Check sheet for the modelled part. Datum: model origin and axes. Units: mm. Face numbers are marked on the shaded views. A direction names the side the tool comes from. Give positions to 0.01 mm unless a question says otherwise; leave off trailing zeros. Write each loop counter-clockwise with the first axis right and the second up, starting at its lowest first coordinate (ties: lowest second). Pieces come first, ordered by that corner, then holes. Notation, with made-up numbers: (-29, 43) -> (-6, 43) arc R14 cw to (-6, 64) -> close; hole circle Ø4 at (59.25, -23.5). An arc over 180 degrees is marked (long way). Answer as a JSON object with one key per item and string values.
from build123d import *

# Parameters (mm, degrees)
SKETCH1_W                                         = 101.6
SKETCH1_H                                         = 100.0125
BOSS_EXTRUDE1_DEPTH                               = 10.16
CBORE_FOR_5_16_SOCKET_HEAD_CAP_SCREW1_D           = 8.2042
CBORE_FOR_5_16_SOCKET_HEAD_CAP_SCREW1_CBORE_D     = 13.49502
CBORE_FOR_5_16_SOCKET_HEAD_CAP_SCREW1_CBORE_DEPTH = 7.9375
SKETCH4_R                                         = 30.1625
BOSS_EXTRUDE2_DEPTH                               = 2.54
CBORE_FOR_3_8_SOCKET_HEAD_CAP_SCREW1_D            = 9.8044
CBORE_FOR_3_8_SOCKET_HEAD_CAP_SCREW1_CBORE_D      = 15.875
CBORE_FOR_3_8_SOCKET_HEAD_CAP_SCREW1_CBORE_DEPTH  = 9.525
FILLET1_R                                         = 2.54


with BuildPart() as part:
    # Sketch1 → Boss-Extrude1 (new body)
    with BuildSketch(Plane.XY):
        with Locations((50.8, 50.00625)):
            Rectangle(SKETCH1_W, SKETCH1_H)
    extrude(amount=BOSS_EXTRUDE1_DEPTH)

    # CBORE for 5/16 Socket Head Cap Screw1 (through all)
    with Locations(Plane.XY.offset(10.16)):
        with Locations((88.9, 8.73125), (88.9, 91.28125), (12.7, 8.73125), (12.7, 91.28125)):
            CounterBoreHole(CBORE_FOR_5_16_SOCKET_HEAD_CAP_SCREW1_D / 2, CBORE_FOR_5_16_SOCKET_HEAD_CAP_SCREW1_CBORE_D / 2, CBORE_FOR_5_16_SOCKET_HEAD_CAP_SCREW1_CBORE_DEPTH)

    # Sketch4 → Boss-Extrude2 (add)
    with BuildSketch(Plane.XY.offset(10.16)):
        with Locations(Location((50.8, 50.00625, 0), (0, 0, 180))):
            Circle(SKETCH4_R)
    extrude(amount=BOSS_EXTRUDE2_DEPTH)

    # CBORE for 3/8 Socket Head Cap Screw1 (through all)
    with Locations(Plane(origin=(0, 0, 0), x_dir=(-1, 0, 0), z_dir=(0, 0, -1))):
        with Locations((-50.8, 50.00625)):
            CounterBoreHole(CBORE_FOR_3_8_SOCKET_HEAD_CAP_SCREW1_D / 2, CBORE_FOR_3_8_SOCKET_HEAD_CAP_SCREW1_CBORE_D / 2, CBORE_FOR_3_8_SOCKET_HEAD_CAP_SCREW1_CBORE_DEPTH)

    # Fillet1
    fillet1_edges = [part.edges().sort_by_distance(p)[0] for p in [
        (0, 100.0125, 5.08),
        (101.6, 100.0125, 5.08),
        (101.6, 0, 5.08),
        (0, 0, 5.08),
    ]]
    fillet(fillet1_edges, radius=FILLET1_R)


solid = part.part
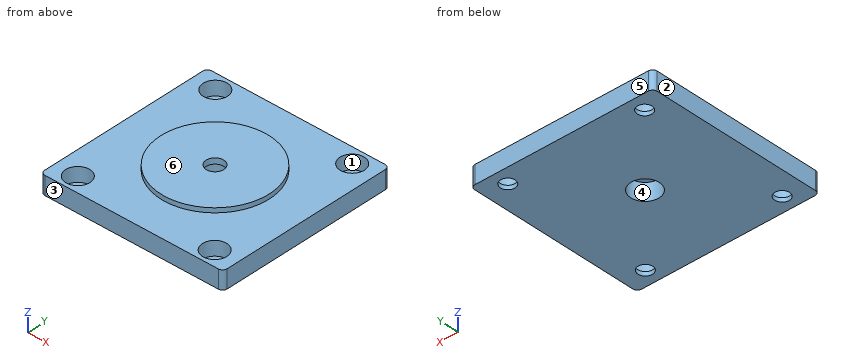
1. Scan lines: L1, parallel to Y at x = 88.9, z = 0.9; L2, parallel to Y at x = 88.9, z = 5.25; L3, parallel to Z at x = 27, y = 77. Record each from-to range of solid material in increasing order. Write a range as [from, to].
Determined:
{"L1": "[0, 4.63], [12.83, 87.18], [95.38, 100.01]", "L2": "[0, 1.98], [15.48, 84.53], [98.03, 100.01]", "L3": "[0, 10.16]"}
2. Mould release check, pull along Y, two halves, no side actions. Record for the marked faces 3, 4, 5 and 6: released by +Y, released by -Y, zero draft, split by the parting line, or undercut.
Determined:
{"face 3": "released by -Y", "face 4": "undercut", "face 5": "released by +Y", "face 6": "zero draft"}
3. Access from +Z, -Z, +X, -X, +Y, -Y to the whole of each face (thin tool, end or side, straight path). Record for the marked faces 1 and 2.
Determined:
{"face 1": "+Z", "face 2": "+Z, -Z, -X, +Y, -Y"}
4. Sectioned sample at B-B, the plane x = 12.7. Enter the section's corners in (y, z), plus the area to 3 significant figures.
Determined:
{"outline": "(0, 0) -> (4.63, 0) -> (4.63, 2.22) -> (1.98, 2.22) -> (1.98, 10.16) -> (0, 10.16) -> close; (12.83, 0) -> (87.18, 0) -> (87.18, 2.22) -> (84.53, 2.22) -> (84.53, 10.16) -> (15.48, 10.16) -> (15.48, 2.22) -> (12.83, 2.22) -> close; (95.38, 0) -> (100.01, 0) -> (100.01, 10.16) -> (98.03, 10.16) -> (98.03, 2.22) -> (95.38, 2.22) -> close", "area": "765 mm^2"}
5. Sectioned sample at A-A, the plane x = 50.8. Enter the section's corners in (y, z) (1 decimal), plus the area to 3 significant figures.
Determined:
{"outline": "(0, 0) -> (42.1, 0) -> (42.1, 9.5) -> (45.1, 9.5) -> (45.1, 12.7) -> (19.8, 12.7) -> (19.8, 10.2) -> (0, 10.2) -> close; (54.9, 9.5) -> (57.9, 9.5) -> (57.9, 0) -> (100, 0) -> (100, 10.2) -> (80.2, 10.2) -> (80.2, 12.7) -> (54.9, 12.7) -> close", "area": "987 mm^2"}
6. Sectioned sample at D-D, the plane z = 5. Enter the section's corners in (x, y) (1 decimal).
Determined:
{"outline": "(0, 2.5) arc R2.5 ccw to (2.5, 0) -> (99.1, 0) arc R2.5 ccw to (101.6, 2.5) -> (101.6, 97.5) arc R2.5 ccw to (99.1, 100) -> (2.5, 100) arc R2.5 ccw to (0, 97.5) -> close; hole circle Ø13.5 at (12.7, 8.7); hole circle Ø13.5 at (12.7, 91.3); hole circle Ø15.9 at (50.8, 50); hole circle Ø13.5 at (88.9, 8.7); hole circle Ø13.5 at (88.9, 91.3)"}
7. Go/stop test with flat-tipped pins: P1, Ø6.5, axis at x = 10.5, y = 91.5, coming from the +Z side; P2, Ø6.5, axis at x = 12.7, y = 91.28, coming from the -Z side; P3, Ø21.5, axis at x = 88.9, y = 8.73, coming from the +Z side. Record where each tip stops, or that it passes through.
Determined:
{"P1": "z = 2.22", "P2": "through", "P3": "z = 10.16"}
8. Sectioned sample at C-C, the plane y = 90. Enter the section's corners in (x, z), plus the area to 3 significant figures.
Determined:
{"outline": "(0, 0) -> (8.8, 0) -> (8.8, 2.22) -> (6.08, 2.22) -> (6.08, 10.16) -> (0, 10.16) -> close; (16.6, 0) -> (85, 0) -> (85, 2.22) -> (82.28, 2.22) -> (82.28, 10.16) -> (19.32, 10.16) -> (19.32, 2.22) -> (16.6, 2.22) -> close; (92.8, 0) -> (101.6, 0) -> (101.6, 10.16) -> (95.52, 10.16) -> (95.52, 2.22) -> (92.8, 2.22) -> close", "area": "787 mm^2"}
